Part print with two shaded views. Sizes in mm from the minimum x, y, z corner. A direction names the side the tool comes from. Coordinates: 2 decimals unless noted, no trailing zeros. Loops run counter-clockwise (first coordinate to the right, second up) from the corner with the lowest first, then second, coordinate; pieces in that order, holes last.
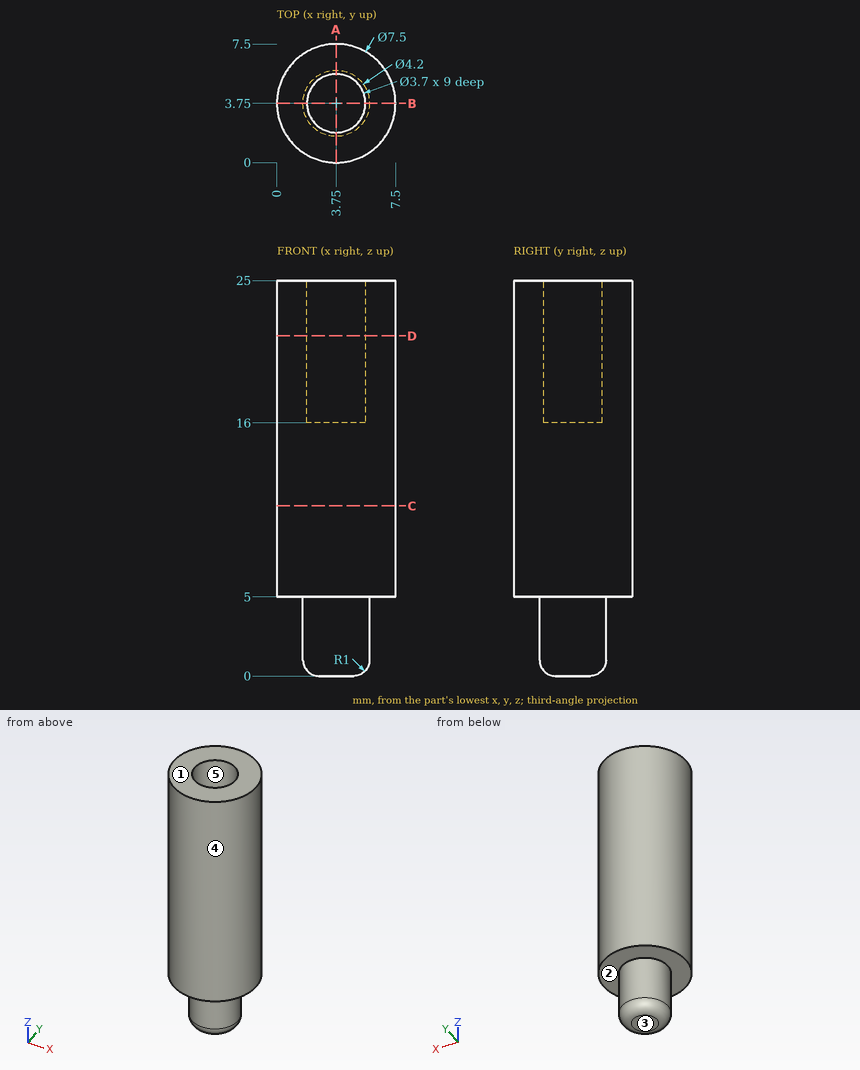
Q1. Drill centre lines: line 1 (Y direction, x = 3.75, z = 20.5); line 2 (Z direction, x = 3.75, y = 6.5); line 3 (X direction, y = 5, z = 18). Where is each one in solid material? Low to high.
Answers:
line 1: y = 0 to 1.9, 5.6 to 7.5
line 2: z = 5 to 25
line 3: x = 0.21 to 2.39, 5.11 to 7.29
Q2. Slice it at C-C (z = 10.75). List the corners of the cut face in (x, y), and give its area (3 significant figures).
Answers:
outline: circle Ø7.5 at (3.75, 3.75)
area: 44.2 mm2
Q3. Slice it at D-D (z = 21.5). List the corners of the cut face in (x, y).
Answers:
outline: circle Ø7.5 at (3.75, 3.75); hole circle Ø3.7 at (3.75, 3.75)
Q4. Flat gauge pin, fed straight in: P1, Ø3, axis at y = 5.5, z = 5.5, coming from the +X side. Where does the tip first touch, or does it go through?
Answers:
P1: stops at x = 7.49
Q5. Which spindle directions (+Z, -Z, +X, -X, +Y, -Y) get a long thin tool onto all of the face, cutting with end or side? Do the marked faces 1 and 2. Say none if no direction does.
Answers:
face 1: +Z, +X, -X, +Y, -Y
face 2: -Z
Q6. Slice it at A-A (x = 3.75). List the corners of the cut face in (y, z), and give its area (3 significant figures).
Answers:
outline: (0, 5) - (1.65, 5) - (1.65, 1) arc R1 ccw to (2.65, 0) - (4.85, 0) arc R1 ccw to (5.85, 1) - (5.85, 5) - (7.5, 5) - (7.5, 25) - (5.6, 25) - (5.6, 16) - (1.9, 16) - (1.9, 25) - (0, 25) - close
area: 137 mm2
Q7. Mould opens along Y. For the marked faces 3, 4 and 5 say: +Y half, -Y half, draft (parallel to the pull), parting line (faces both ways), or undercut.
Answers:
face 3: draft
face 4: parting line
face 5: undercut
